Here's how the part is built. I have some questions about the finished solid (model axes, mm). A direction names the side the tool comes from. Coordinates: 2 decimals unless noted, no trailing zeros. Write each loop counter-clockwise with the first axis right and the second up, starting at its lowest first coordinate (ties: lowest second). Pieces come first, ordered by that corner, then holes. Notation, with made-up numbers: M -20,68.25 L 11,68.25 A10 ccw 11,72.25 Z; hole C -14.5,3 d2. An arc over 180 degrees is marked long. Write each question's results on one line, items separated by ' | '. Start each with the question number.
from build123d import *

# Parameters (mm, degrees)
SKETCH1_W                                        = 50.8
SKETCH1_H                                        = 50.8
BOSS_EXTRUDE1_DEPTH                              = 9.525
TAP_DRILL_FOR_M4X0_7_TAP1_D                      = 3.3
CBORE_FOR_1_4_SOCKET_HEAD_CAP_SCREW1_D           = 6.5278
CBORE_FOR_1_4_SOCKET_HEAD_CAP_SCREW1_CBORE_D     = 9.525
CBORE_FOR_1_4_SOCKET_HEAD_CAP_SCREW1_CBORE_DEPTH = 6.35
FILLET1_R                                        = 2.54


with BuildPart() as part:
    # Sketch1 → Boss-Extrude1 (new body)
    with BuildSketch(Plane.XY):
        with Locations((25.4, 25.4)):
            Rectangle(SKETCH1_W, SKETCH1_H)
    extrude(amount=BOSS_EXTRUDE1_DEPTH)

    # Tap Drill for M4x0.7 Tap1 (through all)
    with Locations(Plane.XY.offset(9.525)):
        with Locations((39.8, 10.4), (39.8, 40.4), (9.8, 40.4), (9.8, 10.4)):
            Hole(TAP_DRILL_FOR_M4X0_7_TAP1_D / 2)

    # CBORE for 1/4 Socket Head Cap Screw1 (through all)
    with Locations(Plane.XY.offset(9.525)):
        with Locations((44.45, 12.7), (44.45, 38.1), (5.08, 12.7), (5.08, 38.1)):
            CounterBoreHole(CBORE_FOR_1_4_SOCKET_HEAD_CAP_SCREW1_D / 2, CBORE_FOR_1_4_SOCKET_HEAD_CAP_SCREW1_CBORE_D / 2, CBORE_FOR_1_4_SOCKET_HEAD_CAP_SCREW1_CBORE_DEPTH)

    # Fillet1
    fillet1_edges = [part.edges().sort_by_distance(p)[0] for p in [
        (0, 50.8, 4.7625),
        (50.8, 50.8, 4.7625),
        (50.8, 0, 4.7625),
        (0, 0, 4.7625),
    ]]
    fillet(fillet1_edges, radius=FILLET1_R)


solid = part.part
1) Please list where these lines run through material, in increasing order: line 1 (Y direction, x = 5.08, z = 7); line 2 (X direction, y = 12.7, z = 7.5); line 3 (Y direction, x = 39.8, z = 3). Write a range as [from, to].
2) I want a section at A-A, the plane y = 38.1. Give the number of separate pieces and of enclosed holes in the cut face, then the cut area to 3 significant figures.
3) We'd pull the mould along X, two halves only. Please class faces 3 (the cylindrical face through (5.505, 41.336, 1.565)), 4 (the flat face through (25, 50.8, 5)), 5 (the cylindrical face through (50.076, 50.036, 4.829)): pulls with the +X half, pulls with the -X half, needs draft (parallel to the pull), parting line crosses it, or undercut.
4) For pin 1 Ø4 at (x, y) = (44.5, 44.5) entering from -Z; pin 2 Ø7.5 at (x, y) = (44.45, 38.1) entering from +Z (3 decimals); pin 3 Ø5.5 at (x, y) = (44.45, 12.7) entering from -Z, each with a flat end and sliding along its axis, tell me the tip position at first contact or that it passes through.
5) For faces 1 (the cylindrical face through (5.788, 9.514, 1.565)), 2 (the flat face through (48, 39, 3.175)), which set-ups out of +Z, -Z, +X, -X, +Y, -Y let a thin tool reach every point of the face, with its end or its side?
6) I want a section at B-B, the plane y = 10.4. Write out the boundary of the cut face in (x, z) (3 decimals).
Output:
1) line 1: y = [0, 7.94], [17.46, 33.34], [42.86, 50.8] | line 2: x = [0, 0.32], [9.84, 39.69], [49.21, 50.8] | line 3: y = [0, 8.75], [12.05, 38.75], [42.05, 50.8]
2) separate pieces: 3 | enclosed holes: 0 | area: 321 mm2
3) face 3: undercut | face 4: needs draft | face 5: pulls with the +X half
4) pin 1: stops at z = 0 | pin 2: stops at z = 3.175 | pin 3: passes through
5) face 1: +Z, -Z | face 2: +Z
6) outline: M 0,0 L 2.764,0 L 2.764,3.175 L 0.91,3.175 L 0.91,9.525 L 0,9.525 Z; M 7.396,0 L 8.15,0 L 8.15,3.175 L 7.396,3.175 Z; M 11.45,0 L 38.15,0 L 38.15,9.525 L 11.45,9.525 Z; M 41.45,0 L 42.134,0 L 42.134,3.175 L 41.45,3.175 Z; M 46.766,0 L 50.8,0 L 50.8,9.525 L 48.62,9.525 L 48.62,3.175 L 46.766,3.175 Z
